Here's how the part is built. I have some questions about the finished solid (model axes, mm). A direction names the side the tool comes from. Round coordinates to 2 decimals unless told otherwise and drop trailing zeros. Loops run counter-clockwise (first coordinate to the right, second up) from the corner with the lowest first, then second, coordinate; pieces in that order, holes last. Notation, with made-up numbers: M 48.5,34 L 71.5,34 A21 cw 71.5,71 Z; hole C 30.25,8.5 d5. An arc over 180 degrees is marked long. Answer as a JSON object with one key per item and string values.
Autodesk Inventor part; units mm, degrees
ref_plane "YZ Plane" through (0, 0, 0) normal (1, 0, 0) x (0, 1, 0)
ref_plane "XZ Plane" through (0, 0, 0) normal (0, 1, 0) x (-1, 0, 0)
ref_plane "XY Plane" through (0, 0, 0) normal (0, 0, 1) x (1, 0, 0)
sketch "Sketch1" plane through (0, 0, 0) normal (0, 0, 1) x (1, 0, 0)
  line L0 (0, 0) -> (88.9, 0)
  line L1 (22.225, 57.15) -> (22.225, 88.9)
  line L2 (22.225, 88.9) -> (66.675, 88.9)
  line L3 (66.675, 88.9) -> (66.675, 57.15)
  line L4 (88.9, 0) -> (88.9, 38.1)
  line L5 (88.9, 38.1) -> (66.675, 57.15)
  line L6 (0, 0) -> (0, 38.1)
  line L7 (0, 38.1) -> (22.225, 57.15)
  line L8 (22.225, 57.15) -> (66.675, 57.15)
  dimension "d4" = 44.45
  dimension "d12" = 38.1
  dimension "d13" = 38.1
  dimension "d14" = 44.45
  dimension "d15" = 31.75
  dimension "d16" = 88.9
extrude "Extrusion1" add sketch "Sketch1" along normal blind 127
sketch "Sketch2" plane through (0, 0, 127) normal (0, 0, 1) x (1, 0, 0)
  line L0 (0, 0) -> (88.9, 0)
  line L1 (44.45, 0) -> (44.45, 19.05)
  circle A0 centre (44.45, 19.05) radius 25.4
  line L2 (19.05, 19.05) -> (19.05, 0)
  line L3 (69.85, 0) -> (69.85, 19.05)
  dimension "d8" = 19.05
  dimension "d9" = 50.8
extrude "Extrusion2" cut sketch "Sketch2" against normal through all
sketch "Sketch3" plane through (0, 0, 127) normal (0, 0, 1) x (1, 0, 0)
  line L0 (22.225, 88.9) -> (34.925, 88.9)
  line L1 (66.675, 88.9) -> (22.225, 88.9)
  line L2 (34.925, 88.9) -> (53.975, 88.9)
  line L3 (53.975, 88.9) -> (66.675, 88.9)
  line L4 (34.925, 88.9) -> (34.925, 57.15)
  line L5 (53.975, 88.9) -> (53.975, 57.15)
  line L6 (53.975, 57.15) -> (34.925, 57.15)
  point P0 (0, 0)
  point P1 (22.225, 57.15)
  point P2 (66.675, 57.15)
  dimension "d17" = 12.7
  dimension "d18" = 19.05
extrude "Extrusion3" cut sketch "Sketch3" against normal through all
sketch "Sketch4" plane through (88.9, 0, 0) normal (1, 0, 0) x (0, 0, -1)
  line L0 (-127, 0) -> (-107.95, 0)
  line L1 (0, 0) -> (-127, 0)
  line L2 (-107.95, 0) -> (-107.95, 56.6372)
  line L3 (-107.95, 56.6372) -> (-19.0515, 57.15)
  line L4 (0, 57.15) -> (-127, 57.15)
  line L5 (-19.0515, 57.15) -> (-18.7218, 0)
  dimension "d21" = 19.05
  dimension "d22" = 88.9
extrude "Extrusion4" cut sketch "Sketch4" against normal through all
sketch "Sketch5" plane through (66.675, 57.15, 0) normal (1, 0, 0) x (0, 0, -1)
  line L0 (0, 31.75) -> (-25.4, 31.75)
  line L1 (0, 31.75) -> (-127, 31.75)
  line L2 (-25.4, 31.75) -> (-25.4, 19.05)
  line L3 (-25.4, 19.05) -> (-101.6, 19.05)
  line L4 (-101.6, 19.05) -> (-101.6, 31.75)
  point P0 (0, -57.15)
  dimension "d25" = 25.4
  dimension "d26" = 12.7
  dimension "d27" = 76.2
extrude "Extrusion5" cut sketch "Sketch5" against normal through all
sketch "Sketch6" plane through (66.675, 57.15, 0) normal (1, 0, 0) x (0, 0, -1)
  line L0 (-101.6, 31.75) -> (-127, 31.75)
  circle A0 centre (-114.3, 31.75) radius 12.7
  point P0 (0, -57.15)
extrude "Extrusion6" add sketch "Sketch6" against normal blind 44.45
sketch "Sketch7" plane through (0, 0, 127) normal (0, 0, 1) x (1, 0, 0)
  line L0 (66.675, 101.6) -> (22.225, 101.6)
  line L1 (34.925, 57.15) -> (53.975, 57.15)
  line L2 (53.975, 57.15) -> (53.975, 101.6)
  line L3 (53.975, 101.6) -> (34.925, 101.6)
  line L4 (34.925, 101.6) -> (34.925, 57.15)
  point P0 (0, 0)
extrude "Extrusion7" cut sketch "Sketch7" against normal blind 44.45
sketch "Sketch8" plane through (66.675, 57.15, 0) normal (1, 0, 0) x (0, 0, -1)
  line L0 (-127, 31.75) -> (-101.7646, 31.75)
  circle A0 centre (-114.3823, 31.75) radius 6.35
  point P0 (0, -57.15)
  dimension "d34" = 12.7
extrude "Extrusion8" cut sketch "Sketch8" against normal through all
properties part number "3-4"
Item 1: If I drill on L1, parallel to Z at x = 45.5, y = 44.5; L2, parallel to Z at x = 32, y = 88; L3, parallel to X at y = 62.5, z = 108.5 (3 decimals), over which ranges is the centre line in solid material (lowest first)? Write a range as from..to.
Solution:
{"L1": "z = 0..18.98, 107.95..127", "L2": "z = 0..25.4, 101.6..108.1, 120.67..127", "L3": "x = 22.225..34.925, 53.975..66.675"}
Item 2: I want a section at C-C on y = 6.5. List the corners of the cut face in (x, z) for me.
Solution:
{"outline": "M 0,0 L 19.05,0 L 19.05,18.76 L 0,18.76 Z; M 0,107.95 L 19.05,107.95 L 19.05,127 L 0,127 Z; M 69.85,0 L 88.9,0 L 88.9,18.76 L 69.85,18.76 Z; M 69.85,107.95 L 88.9,107.95 L 88.9,127 L 69.85,127 Z"}
Item 3: I want a section at D-D on y = 54. List the corners of the cut face in (x, z) for me, plus the area to 3 significant figures.
Solution:
{"outline": "M 18.55,0 L 70.35,0 L 70.35,19.03 L 18.55,19.03 Z; M 18.55,107.95 L 70.35,107.95 L 70.35,127 L 18.55,127 Z", "area": "1,970 mm2"}
Item 4: For faces 1 (the face through (69.85, 9, 118)), 2 (the face through (34.925, 75, 64)), 3 (the face through (66.675, 70, 63)), 4 (the face through (60, 76.2, 63)), 5 (the face through (28, 88.9, 13)), which set-ups out of +Z, -Z, +X, -X, +Y, -Y let a thin tool reach every point of the face, with its end or its side?
Solution:
{"face 1": "+Z, -Z, -Y", "face 2": "+Z, -Z, +Y", "face 3": "+Z, -Z, +X, +Y", "face 4": "+X, -X, +Y", "face 5": "-Z, +X, -X, +Y"}
Item 5: We'd pull the mould along X, two halves only. Please class faces 6 (the face through (88.9, 19, 117)), 7 (the face through (10.957, 47.492, 9.392)), 8 (the face through (19.05, 10, 10)): +X half, -X half, draft (parallel to the pull), parting line (faces both ways), or undercut.
Solution:
{"face 6": "+X half", "face 7": "-X half", "face 8": "undercut"}
Item 6: I want a section at B-B on z = 114.3. List the corners of the cut face in (x, y) for me (3 decimals), plus the area to 3 significant figures.
Solution:
{"outline": "M 0,0 L 19.05,0 L 19.05,19.05 A25.4 cw 69.85,19.05 L 69.85,0 L 88.9,0 L 88.9,38.1 L 66.675,57.15 L 66.675,82.551 L 53.975,82.551 L 53.975,57.15 L 34.925,57.15 L 34.925,82.551 L 22.225,82.551 L 22.225,57.15 L 0,38.1 Z; M 22.225,95.249 L 34.925,95.249 L 34.925,101.6 L 22.225,101.6 Z; M 53.975,95.249 L 66.675,95.249 L 66.675,101.6 L 53.975,101.6 Z", "area": "3,480 mm2"}
Item 7: For P1, Ø4, axis at x = 32, z = 93, coming from the -Y side; P2, Ø10, axis at x = 30, z = 7.5, coming from the +Y side; P3, Ø14, axis at x = 62.5, z = 74.5, coming from the +Y side, each with a flat end and sliding along its axis, tell me the tip position at first contact or that it passes through.
Solution:
{"P1": "stops at y = 56.71", "P2": "stops at y = 88.9", "P3": "stops at y = 76.2"}
